```python
from build123d import *

# Parameters (mm, degrees)
SKETCH7_W           = 40
SKETCH7_H           = 40
BOSS_EXTRUDE1_DEPTH = 14
LOFT1_START         = -20
LOFT1_DEPTH         = 40
SKETCH16_W          = 49.026286786
SKETCH16_H          = 65.242270374
SKETCH16_R          = 20
CUT_EXTRUDE3_DEPTH  = 6
SKETCH17_W          = 40
SKETCH17_H          = 8
BOSS_EXTRUDE5_DEPTH = 230
SKETCH10_R          = 2.25
CUT_EXTRUDE1_DEPTH  = 25
CHAMFER1_SIZE       = 2.5
FILLET3_R           = 20
FILLET4_R           = 20
SKETCH41_R          = 2.55
CUT_EXTRUDE4_DEPTH  = 20
LPATTERN1_COUNT     = 15
LPATTERN1_PITCH     = 10


# Read off the part's stored shape, not the designer's step: Loft1
with BuildPart() as part:
    # Sketch7 → Boss-Extrude1 (new body)
    with BuildSketch(Plane.XY):
        Rectangle(SKETCH7_W, SKETCH7_H)
    extrude(amount=BOSS_EXTRUDE1_DEPTH)

    # Loft1 outline → Loft1 (add)
    with BuildSketch(Plane.YZ.offset(LOFT1_START)):
        with BuildLine():
            add(Edge.make_bspline(
                [(-38, 18), (-31.853637028, 18), (-26.146362972, 14), (-20, 14)],
                knots=[0, 0, 0, 0, 1, 1, 1, 1], degree=3))
            Line((-38, 18), (-38, 10))
            add(Edge.make_bspline(
                [(-38, 10), (-31.853637028, 10), (-26.146362972, 6), (-20, 6)],
                knots=[0, 0, 0, 0, 1, 1, 1, 1], degree=3))
            Line((-20, 6), (-20, 14))
        make_face()
    extrude(amount=LOFT1_DEPTH)

    # Sketch16 → Cut-Extrude3 (cut)
    with BuildSketch(Plane(origin=(0, 0, 0), x_dir=(-1, 0, 0), z_dir=(0, 0, -1))):
        Rectangle(SKETCH16_W, SKETCH16_H)
        Circle(SKETCH16_R, mode=Mode.SUBTRACT)
    extrude(amount=-CUT_EXTRUDE3_DEPTH, mode=Mode.SUBTRACT)

    # Sketch17 → Boss-Extrude5 (add)
    with BuildSketch(Plane(origin=(0, -38, 0), x_dir=(-1, 0, 0), z_dir=(0, -1, 0))):
        with Locations((0, -14)):
            Rectangle(SKETCH17_W, SKETCH17_H)
    extrude(amount=BOSS_EXTRUDE5_DEPTH)

    # Sketch10 → Cut-Extrude1 (cut)
    with BuildSketch(Plane.XY.offset(14)):
        with Locations((-7.00009521, 12.124420806)):
            Circle(SKETCH10_R)
        with Locations((6.99990479, 12.124420806)):
            Circle(SKETCH10_R)
        with Locations((13.99990479, 6.5153e-05)):
            Circle(SKETCH10_R)
        with Locations((6.99990479, -12.1242905)):
            Circle(SKETCH10_R)
        with Locations((-7.00009521, -12.1242905)):
            Circle(SKETCH10_R)
        with Locations((-14.00009521, 6.5153e-05)):
            Circle(SKETCH10_R)
    extrude(amount=-CUT_EXTRUDE1_DEPTH, mode=Mode.SUBTRACT)

    # Chamfer1
    chamfer1_edges = [part.edges().sort_by_distance(p)[0] for p in [
        (4.74990479, 12.124420806, 14),
        (-9.25009521, 12.124420806, 14),
        (-16.25009521, 6.5153e-05, 14),
        (-9.25009521, -12.1242905, 14),
        (4.74990479, -12.1242905, 14),
        (11.74990479, 6.5153e-05, 14),
    ]]
    chamfer(chamfer1_edges, length=CHAMFER1_SIZE)

    # Fillet3
    fillet3_edges = [part.edges().sort_by_distance(p)[0] for p in [
        (20, 20, 10),
        (-20, 20, 10),
    ]]
    fillet(fillet3_edges, radius=FILLET3_R - 0.0001)  # a hair under: the kernel refuses the full size

    # Fillet4
    fillet4_edges = [part.edges().sort_by_distance(p)[0] for p in [
        (-20, -268, 14),
        (20, -268, 14),
    ]]
    fillet(fillet4_edges, radius=FILLET4_R - 0.0001)  # a hair under: the kernel refuses the full size

    # Sketch41 → Cut-Extrude4 (cut)
    with BuildSketch(Plane.XY):
        with Locations(Location((0, -258, 0), (0, 0, 180))):
            Circle(SKETCH41_R)
    cut_extrude4 = extrude(amount=CUT_EXTRUDE4_DEPTH, mode=Mode.SUBTRACT)

    # LPattern1: Cut-Extrude4 ×15
    with Locations(*[(0, i * LPATTERN1_PITCH, 0) for i in range(1, LPATTERN1_COUNT)]):
        add(cut_extrude4, mode=Mode.SUBTRACT)


solid = part.part
```
Work out the finished part from the listing and answer in its coordinate system (mm). A direction names the side the tool comes from. Round coordinates to 2 decimals unless told otherwise and drop trailing zeros. Loops run counter-clockwise (first coordinate to the right, second up) from the corner with the lowest first, then second, coordinate; pieces in that order, holes last. Notation, with made-up numbers: (81.5, -12) -> (93.5, -12) arc R11 ccw to (93.5, 0) -> close; hole circle Ø1 at (-35, -11). An arc over 180 degrees is marked (long way). Write each question's results on one line, items separated by ' | '. Start each with the question number.
1. Find the intervals of material crossed by probe 1 along X at (y, z) = (-128.5, 13.75); probe 2 along Y at (x, z) = (6.5, 1.75); probe 3 along X at (y, z) = (1, 8), in increasing order. Write a range as from..to.
2. Section A-A (y = -188) is taken. Determine the outline of the cut face in (x, z), plus the area to 3 significant figures.
3. A tool of negligible diameter and unlimited length cuts with its end or side. For faces 1 (the face through (14.297, -261.986, 13.944)), 2 (the face through (-16, -16, 6)), from which of +Z, -Z, +X, -X, +Y, -Y can it reach the whole face along a straight path? Write none if from no direction.
4. Section B-B (y = -45) is taken. Determine the outline of the cut face in (x, z).
5. For a pull along X with two mould halves and no side action, classify faces 3 (the face through (13.986, 14.297, 10.056)), 4 (the face through (0, -151, 10)), 5 (the face through (0.33, -200.53, 13.94)) as +X half, -X half, draft (parallel to the pull), parting line (faces both ways), or undercut.
6. Section C-C (y = -258) is taken. Determine the outline of the cut face in (x, z).
7. Given pin 1 Ø1.5 at (x, z) = (-5.5, 12.5) entering from +Y; pin 2 Ø3 at (x, y) = (0, -208) entering from +Z; pin 3 Ø2 at (x, z) = (12.5, 3.5) entering from -Y; pin 4 Ø6 at (x, z) = (-2.5, 16) entering from +Y, each flat-ended and moving along its own axis, determine where each tip first touches the part or whether it passes through.
Evaluation:
1) probe 1: x = -20..-2.5, 2.5..20 | probe 2: y = -18.91..-14.32, -9.93..9.93, 14.32..18.91 | probe 3: x = -19.97..-16.02, -11.98..11.98, 16.02..19.97
2) outline: (-20, 10) -> (-2.55, 10) -> (-2.55, 18) -> (-20, 18) -> close; (2.55, 10) -> (20, 10) -> (20, 18) -> (2.55, 18) -> close | area: 279 mm2
3) face 1: +Z, -Z, +X, -Y | face 2: -Z, -X, -Y
4) outline: (-20, 10) -> (20, 10) -> (20, 18) -> (-20, 18) -> close
5) face 3: +X half | face 4: draft | face 5: undercut
6) outline: (-17.32, 10) -> (-2.55, 10) -> (-2.55, 18) -> (-17.32, 18) -> close; (2.55, 10) -> (17.32, 10) -> (17.32, 18) -> (2.55, 18) -> close
7) pin 1: stops at y = 19.43 | pin 2: passes through | pin 3: stops at y = -16.36 | pin 4: stops at y = 20
